from build123d import *

# Parameters (mm, degrees)
SKETCH_R     = 1.65
PAD_DEPTH    = 17.5
SKETCH001_R  = 1.6
POCKET_DEPTH = 5
CHAMFER_SIZE = 2


with BuildPart() as part:
    # Sketch → Pad (new body)
    with BuildSketch(Plane.XY):
        with BuildLine():
            Line((0, 0), (2.5, 0))
            Line((2.5, 0), (2.5, 11))
            Line((2.5, 11), (4.999996, 11))
            ThreePointArc((4.999996, 11), (8.535546, 19.535522), (0, 16.000029))
            Line((0, 16.000029), (0, 0))
        make_face()
        with Locations((5, 16)):
            Circle(SKETCH_R, mode=Mode.SUBTRACT)
    extrude(amount=PAD_DEPTH)

    # Sketch001 → Pocket (cut)
    with BuildSketch(Plane.YZ.offset(2.5)):
        with Locations((5, 13.5)):
            Circle(SKETCH001_R)
        with Locations((5, 4)):
            Circle(SKETCH001_R)
    extrude(amount=-POCKET_DEPTH, mode=Mode.SUBTRACT)

    # Chamfer
    chamfer_edges = [part.edges().sort_by_distance(p)[0] for p in [
        (1.25, 0, 17.5),
        (1.25, 0, 0),
    ]]
    chamfer(chamfer_edges, length=CHAMFER_SIZE)


solid = part.part
Input: part model. Units: mm. Frame: model coordinates. A direction names the side the tool comes from. Coordinates: 2 decimals unless noted, no trailing zeros. Write each loop counter-clockwise with the first axis right and the second up, starting at its lowest first coordinate (ties: lowest second). Pieces come first, ordered by that corner, then holes. Notation, with made-up numbers: M 32,67 L 52,67 A24 ccw 52,94 Z; hole C -11,-34.5 d11. An arc over 180 degrees is marked long. Answer as a JSON object with one key per item and string values. Group by question number.
(1) Set-up query: faces 1 (the face through (0, 8, 9)), 2 (the face through (2.5, 5, 9)). Return all of +Z, -Z, +X, -X, +Y, -Y with unobstructed straight access to the full face (end or side cutting, diameter ignored); none if empty.
(2) Section C-C on z = 7.25. Output: boundary loops of the cut face in (x, y).
(3) Section D-D on x = 4.75. Output: boundary loops of the cut face in (y, z), plus the area to 3 significant figures.
(4) Contact query for flat-ended pins moving along their axis: P1, Ø9, axis at y = 3.5, z = 5, coming from the +X side; P2, Ø0.7, axis at x = 3.5, z = 5.5, coming from the -Y side. Output: stop coordinate, or through.
(5) Ray query, line 1 along Z through (x, y) = (1.3, 5); line 2 along Y through (x, z) = (5, 9); line 3 along X through (y, z) = (3.5, 12.5). Return the intervals inside material, ascending. Write a range as [from, to].
(6) Section A-A on z = 13.5. Output: boundary loops of the cut face in (x, y), plus the area to 3 significant figures.
(7) Section B-B on y = 14.75. Output: boundary loops of the cut face in (x, z).
(8) Mould query, pull axis Y, two halves, no side actions, for faces 3 (the face through (4, 11, 9)), 4 (the face through (1.268, 4.792, 15.086)), 5 (the face through (9, 19, 9)), 6 (the face through (4, 14, 0)). Classes: pulls with the +Y half, pulls with the -Y half, needs draft (parallel to the pull), parting line crosses it, or undercut.
Result set:
{
 "1": {"face 1": "+Z, -Z, -X, +Y, -Y", "face 2": "+Z, -Z, +X, -Y"},
 "2": {"outline": "M 0,0 L 2.5,0 L 2.5,11 L 5,11 A5 ccw long 0,16 Z; hole C 5,16 d3.3"},
 "3": {"outline": "M 11,0 L 14.37,0 L 14.37,17.5 L 11,17.5 Z; M 17.63,0 L 20.99,0 L 20.99,17.5 L 17.63,17.5 Z", "area": "118 mm2"},
 "4": {"P1": "stops at x = 2.5", "P2": "stops at y = 11"},
 "5": {"line 1": "z = [0, 2.4], [5.6, 11.9], [15.1, 17.5]", "line 2": "y = [11, 14.35], [17.65, 21]", "line 3": "x = [0, 2.5]"},
 "6": {"outline": "M 0,0 L 2.5,0 L 2.5,3.4 L 0,3.4 Z; M 0,6.6 L 2.5,6.6 L 2.5,11 L 5,11 A5 ccw long 0,16 Z; hole C 5,16 d3.3", "area": "94.9 mm2"},
 "7": {"outline": "M 0,0 L 3.92,0 L 3.92,17.5 L 0,17.5 Z; M 6.08,0 L 9.84,0 L 9.84,17.5 L 6.08,17.5 Z"},
 "8": {"face 3": "pulls with the -Y half", "face 4": "undercut", "face 5": "parting line crosses it", "face 6": "needs draft"}
}
